Study the drawing (mm; zero at the part's minimum x, y, z) and answer. A direction names the side the tool comes from. Round coordinates to 2 decimals unless told otherwise and drop trailing zeros. Write each loop counter-clockwise with the first axis right and the second up, starting at its lowest first coordinate (ties: lowest second). Pieces come first, ordered by that corner, then holes.
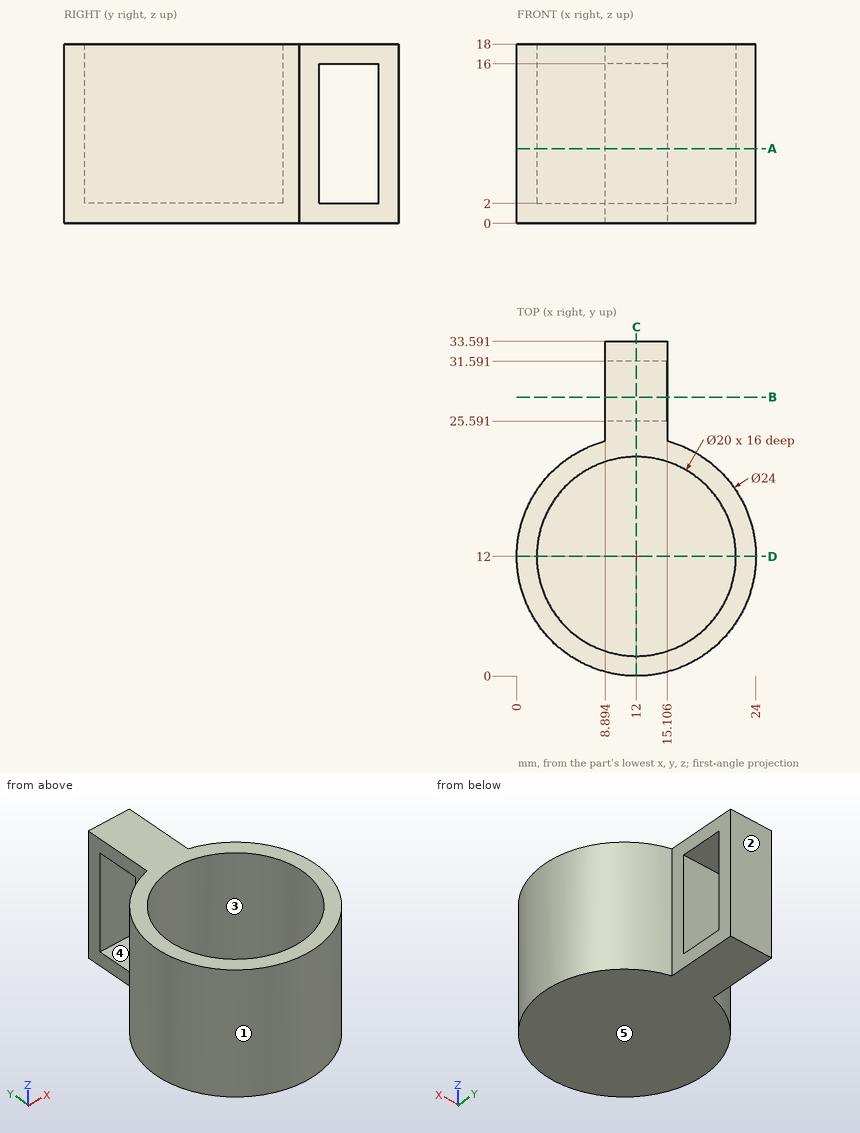
1. Section D-D on y = 12 is taken. Determine the outline of the cut face in (x, z), plus the area to 3 significant figures.
Geometry says:
outline: (0, 0) - (24, 0) - (24, 18) - (22, 18) - (22, 2) - (2, 2) - (2, 18) - (0, 18) - close
area: 112 mm2
2. Section C-C on x = 12 is taken. Determine the outline of the cut face in (y, z), plus the area to 3 significant figures.
Geometry says:
outline: (0, 0) - (33.59, 0) - (33.59, 18) - (22, 18) - (22, 2) - (2, 2) - (2, 18) - (0, 18) - close; hole (25.59, 2) - (31.59, 2) - (31.59, 16) - (25.59, 16) - close
area: 201 mm2
3. A tool of negligible diameter and unlimited length cuts with its end or side. For the marked faces 4 and 5, from which of +Z, -Z, +X, -X, +Y, -Y can it reach the whole face along a straight path? Write none if from no direction.
Geometry says:
face 4: +X, -X
face 5: -Z, +X, -X, +Y, -Y
4. Section A-A on z = 7.5 is taken. Determine the outline of the cut face in (x, y), plus the area to 3 significant figures.
Geometry says:
outline: (8.89, 23.59) arc R12 ccw (long way) to (15.11, 23.59) - (15.11, 25.59) - (8.89, 25.59) - close; (8.89, 31.59) - (15.11, 31.59) - (15.11, 33.59) - (8.89, 33.59) - close; hole circle Ø20 at (12, 12)
area: 161 mm2
5. For a pull along Y with two mould halves and no side action, classify the marked faces 1, 2 and 3 as released by +Y, released by -Y, zero draft, split by the parting line, or undercut.
Geometry says:
face 1: split by the parting line
face 2: released by +Y
face 3: undercut
6. Given pin 1 (3 mm diameter, centred on y = 29, z = 4.5, fed in from +X); pin 2 (6 mm diameter, centred on y = 18, z = 10.5, fed in from +X); pin 3 (1 mm diameter, centred on x = 3, z = 11, fed in from -Y); pin 4 (5 mm diameter, centred on x = 19, z = 9, fed in from -Y), each flat-ended and moving along its own axis, determine where each tip first touches the part or whether it passes through.
Geometry says:
pin 1: passes through
pin 2: stops at x = 23.62
pin 3: stops at y = 3.53
pin 4: stops at y = 0.88
7. Straight lines are drawn through the part: line 1 along Y through (x, z) = (12, 14.25); line 2 along Y through (x, z) = (10.5, 4.75); line 3 along X through (y, z) = (12, 7.75). For each, find the intervals that lie inside material, in ascending order.
Geometry says:
line 1: y = 0 to 2, 22 to 25.59, 31.59 to 33.59
line 2: y = 0.09 to 2.11, 21.89 to 25.59, 31.59 to 33.59
line 3: x = 0 to 2, 22 to 24
8. Section B-B on y = 28 is taken. Determine the outline of the cut face in (x, z).
Geometry says:
outline: (8.89, 0) - (15.11, 0) - (15.11, 2) - (8.89, 2) - close; (8.89, 16) - (15.11, 16) - (15.11, 18) - (8.89, 18) - close
